```python
from build123d import *

# Parameters (mm, degrees)
SKETCH_4_W                  = 500
SKETCH_4_H                  = 500
EXTRUDE_2_DEPTH             = 25
SKETCH_9_R                  = 112.5
CUT_EXTRUDE_2_DEPTH         = 100
HOLE_WIZARD_1_4_28_2_D      = 5.4102
PATTERN_CIRCULAR_3_COUNT    = 4
M6X1_0_2_D                  = 5
PATTERN_CIRCULAR_4_COUNT    = 4
HOLE_WIZARD_M10_3_D         = 12
PATTERN_LINEAR_1_COUNT      = 5
PATTERN_LINEAR_1_PITCH      = 100
PATTERN_LINEAR_1_COUNT_DIR2 = 5
PATTERN_LINEAR_1_PITCH_DIR2 = 100
PATTERN_CIRCULAR_5_COUNT    = 4


with BuildPart() as part:
    # ｽｹｯﾁ4 → ﾎﾞｽ - 押し出し2 (new body)
    with BuildSketch(Plane.XY):
        Rectangle(SKETCH_4_W, SKETCH_4_H)
    extrude(amount=EXTRUDE_2_DEPTH)

    # ｽｹｯﾁ9 → ｶｯﾄ - 押し出し2 (cut)
    with BuildSketch(Plane.XY.offset(25)):
        Circle(SKETCH_9_R)
    extrude(amount=-CUT_EXTRUDE_2_DEPTH, mode=Mode.SUBTRACT)

    # 1/4-28 ねじ穴2 (through all)
    with Locations(Plane(origin=(125.365916841, 51.416309616, 25), x_dir=(1, 0, 0), z_dir=(0, 0, 1))):
        with Locations((0, 0), (0, -102.832619232)):
            hole_wizard_1_4_28_2 = Hole(HOLE_WIZARD_1_4_28_2_D / 2)

    # 円形ﾊﾟﾀｰﾝ3: 1/4-28 ねじ穴2 ×4 about axis
    pattern_circular_3_axis = Axis((0, 0, 0), (0, 0, 1))
    for i in range(1, PATTERN_CIRCULAR_3_COUNT):
        add(hole_wizard_1_4_28_2.rotate(pattern_circular_3_axis, i * 360 / PATTERN_CIRCULAR_3_COUNT), mode=Mode.SUBTRACT)

    # M6x1.0 ねじ穴2 (through all)
    with Locations(Plane(origin=(96.146834801, 95.47793545, 25), x_dir=(1, 0, 0), z_dir=(0, 0, 1))):
        with Locations((0, 0), (39.352339687, -95.004952183)):
            m6x1_0_2 = Hole(M6X1_0_2_D / 2)

    # 円形ﾊﾟﾀｰﾝ4: M6x1.0 ねじ穴2 ×4 about axis
    pattern_circular_4_axis = Axis((0, 0, 0), (0, 0, 1))
    for i in range(1, PATTERN_CIRCULAR_4_COUNT):
        add(m6x1_0_2.rotate(pattern_circular_4_axis, i * 360 / PATTERN_CIRCULAR_4_COUNT), mode=Mode.SUBTRACT)

    # M10 すきま穴3 (through all)
    with Locations(Plane(origin=(200, 200, 0), x_dir=(-1, 0, 0), z_dir=(0, 0, -1))):
        with Locations((0, 0)):
            hole_wizard_m10_3 = Hole(HOLE_WIZARD_M10_3_D / 2)

    # 直線ﾊﾟﾀｰﾝ1: Hole Wizard M10 _3 5 × 5, 9 skipped
    with Locations(*[(-i * PATTERN_LINEAR_1_PITCH, -j * PATTERN_LINEAR_1_PITCH_DIR2, 0) for i in range(PATTERN_LINEAR_1_COUNT) for j in range(PATTERN_LINEAR_1_COUNT_DIR2) if (i, j) not in ((0, 0), (1, 1), (1, 2), (1, 3), (2, 1), (2, 2), (2, 3), (3, 1), (3, 2), (3, 3))]):
        add(hole_wizard_m10_3, mode=Mode.SUBTRACT)

    # ｽｹｯﾁ27 → M5x0.8 ねじ穴2 (revolve, cut)
    with BuildSketch(Plane(origin=(-250, 0, 12.5), x_dir=(0, 0, 1), z_dir=(0, 1, 0))):
        Polygon((0, 0), (0, 9.2618073), (2.1, 8), (2.1, 0), align=None)
    m5x0_8_2 = revolve(axis=Axis((-256.35, 0, 12.5), (1, 0, 0)), mode=Mode.SUBTRACT)

    # 円形ﾊﾟﾀｰﾝ5: M5x0.8 ねじ穴2 ×4 about axis
    pattern_circular_5_axis = Axis((0, 0, -171.019585974), (0, 0, 1))
    for i in range(1, PATTERN_CIRCULAR_5_COUNT):
        add(m5x0_8_2.rotate(pattern_circular_5_axis, i * 360 / PATTERN_CIRCULAR_5_COUNT), mode=Mode.SUBTRACT)


solid = part.part
```
Here's how the part is built. I have some questions about the finished solid (model axes, mm). Give positions to 0.01 mm unless a question says otherwise; leave off trailing zeros. Loops run counter-clockwise (first coordinate to the right, second up) from the corner with the lowest first, then second, coordinate; pieces in that order, holes last. Notation, with made-up numbers: M 81.25,-38.75 L 86.25,-38.75 A26 cw 86.25,-4.75 Z; hole C 28.25,31.5 d9. An arc over 180 degrees is marked long. Return JSON: item names as keys, results as strings.
Item 1: Imagine slicing it at A-A on y = 200. List the corners of the cut face in (x, z) for me.
A:
{"outline": "M -250,0 L -206,0 L -206,25 L -250,25 Z; M -194,0 L -106,0 L -106,25 L -194,25 Z; M -94,0 L -6,0 L -6,25 L -94,25 Z; M 6,0 L 94,0 L 94,25 L 6,25 Z; M 106,0 L 194,0 L 194,25 L 106,25 Z; M 206,0 L 250,0 L 250,25 L 206,25 Z"}
Item 2: I'm going to push flat-ended pins straight in: pin 1 Ø4 at (x, y) = (96.15, 95.48) entering from -Z; pin 2 Ø4 at (y, z) = (0, 12.5) entering from -X; pin 3 Ø2.5 at (x, z) = (0, 12.5) entering from -Y; pin 4 Ø3.5 at (y, z) = (0, 12.5) entering from -X. Where does each tip first touch, or does it pass through?
A:
{"pin 1": "passes through", "pin 2": "stops at x = -241.94", "pin 3": "stops at y = -241.49", "pin 4": "stops at x = -241.79"}
Item 3: Thinking about a two-plate mould opening in X: for faces 1 (the flat face through (-250, -3, 12)), 2 (the flat face through (-3, -250, 12)), 3 (the cylindrical face through (98.699, -205.857, 12.675)), which applies, released by +X, released by -X, zero draft, split by the parting line, or undercut?
A:
{"face 1": "released by -X", "face 2": "zero draft", "face 3": "undercut"}
Item 4: Please list where these lines run through material, in increasing order: line 1 (Z direction, x = -245, y = 0); line 2 (Y direction, x = 244.25, z = 12.5); line 3 (Y direction, x = 100, z = 14.25).
A:
{"line 1": "z = 0 to 10.4, 14.6 to 25", "line 2": "y = -250 to -2.1, 2.1 to 250", "line 3": "y = -250 to -206, -194 to -51.54, 51.54 to 194, 206 to 250"}
Item 5: Imagine slicing it at C-C on y = -72.5. List the corners of the cut face in (x, z) for me.
A:
{"outline": "M -250,0 L -86.02,0 L -86.02,25 L -250,25 Z; M 86.02,0 L 250,0 L 250,25 L 86.02,25 Z"}
Item 6: Imagine slicing it at B-B on x = -70.5. List the corners of the cut face in (y, z) for me.
A:
{"outline": "M -250,0 L -87.67,0 L -87.67,25 L -250,25 Z; M 87.67,0 L 250,0 L 250,25 L 87.67,25 Z"}
